Geometry: see drawing. Coordinates: mm, zero at the bounding-box minimum. A direction names the side the tool comes from. Give positions to 0.01 mm unless a question says otherwise; leave off trailing zeros. Write each loop counter-clockwise with the first axis right and the second up, starting at its lowest first coordinate (ties: lowest second). Pieces come first, ordered by that corner, then holes. Notation, with made-up numbers: M -17,-25.5 L 16,-25.5 A35 cw 16,11.5 Z; hole C 47.25,6 d10. An arc over 180 degrees is marked long. Use a Markdown table: item, result. Add a question column.
(1) Cut plane C-C (z = 24). Output: boundary loops of the cut face in (x, y), plus the area to 3 significant figures.
(2) Cut plane D-D (y = 4.25). State how many separate pieces and enclosed holes the cut face has, plus the area to 3 significant figures.
(3) Pin query (flat end, axial travel): pin 1 Ø14.5 at (x, z) = (15, 17) entering from -Y; pin 2 Ø1 at (y, z) = (4, 26) entering from +X. Return the tip coordinate at first contact, or that it passes through.
(4) Draft query along Z for the marked faces 3, 4, 5 and 6. Return one class per face: released by +Z, released by -Z, zero draft, split by the parting line, or undercut.
(5) Cut plane A-A (y = 0.9). Output: boundary loops of the cut face in (x, z).
(6) Reachability of the marked faces 1 and 2 from +Z, -Z, +X, -X, +Y, -Y: full face, straight path, thin tool, end or side. Return the list, or none.
(7) Material intervals for L1, parallel to X at y = 4.5, z = 20; L2, parallel to Z at x = 6, y = 1.7, sorted ascending.
(8) Cut plane B-B (x = 23). Output: boundary loops of the cut face in (y, z).
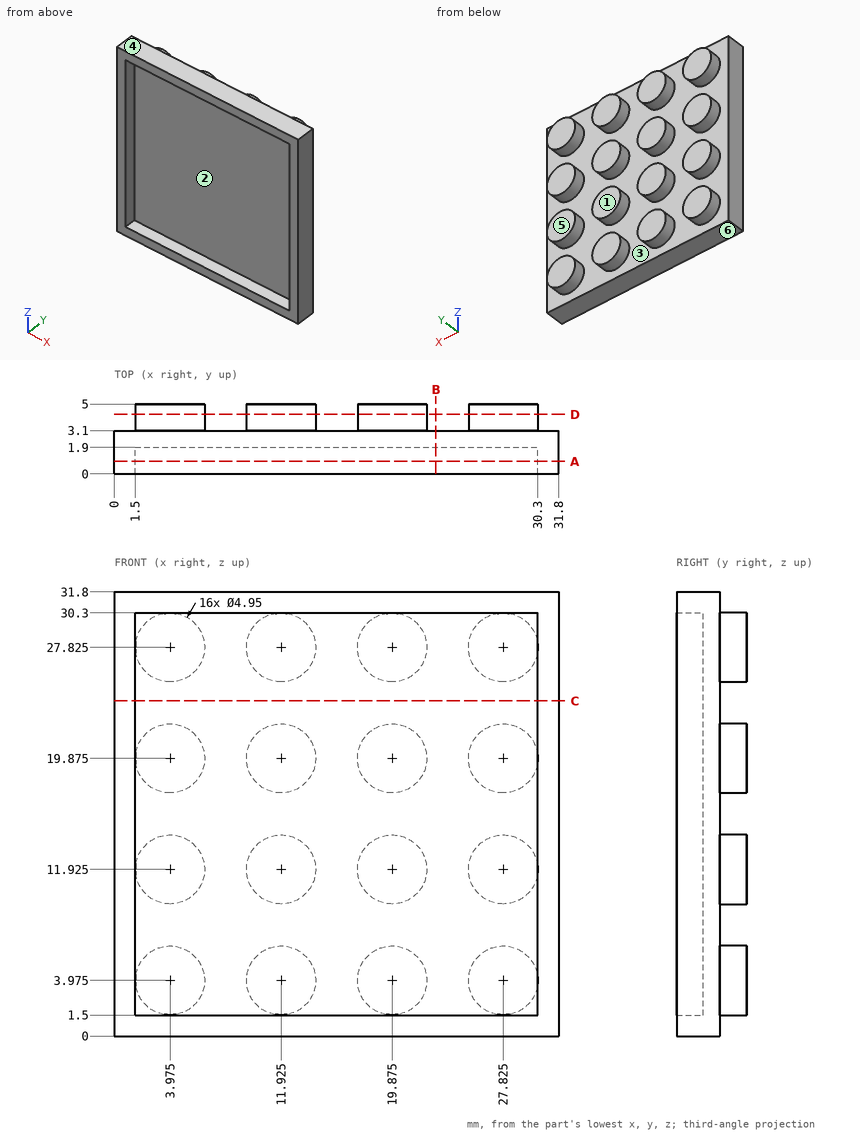
Answer list:
| question | item | result |
|---|---|---|
| 1 | outline | M 0,0 L 1.5,0 L 1.5,1.9 L 30.3,1.9 L 30.3,0 L 31.8,0 L 31.8,3.1 L 0,3.1 Z |
| 1 | area | 43.9 mm² |
| 2 | separate pieces | 16 |
| 2 | enclosed holes | 0 |
| 2 | area | 308 mm² |
| 3 | pin 1 | y = 1.9 |
| 3 | pin 2 | x = 29.92 |
| 4 | face 3 | undercut |
| 4 | face 4 | released by +Z |
| 4 | face 5 | zero draft |
| 4 | face 6 | released by -Z |
| 5 | outline | M 0,0 L 31.8,0 L 31.8,31.8 L 0,31.8 Z; hole M 1.5,1.5 L 30.3,1.5 L 30.3,30.3 L 1.5,30.3 Z |
| 6 | face 1 | +Z, -Z, +X, -X, +Y |
| 6 | face 2 | -Y |
| 7 | L1 | 1.5 to 6.45, 9.45 to 14.4, 17.4 to 22.35, 25.35 to 30.3 |
| 7 | L2 | 0 to 1.5, 30.3 to 31.8 |
| 8 | outline | M 0,0 L 3.1,0 L 3.1,31.8 L 0,31.8 L 0,30.3 L 1.9,30.3 L 1.9,1.5 L 0,1.5 Z |
